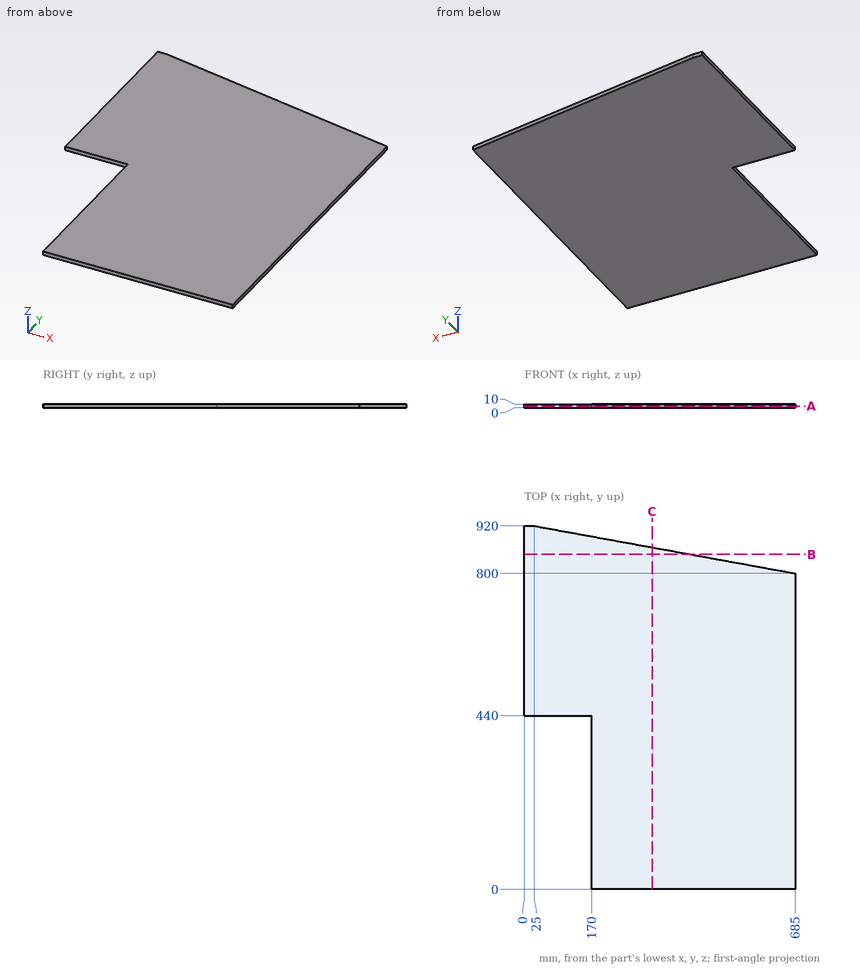
Can you work these out from the drawing? Everything is in mm from the part's minimum corner. Give positions to 0.01 mm unless a question says otherwise; leave off trailing zeros. Loops run counter-clockwise (first coordinate to the right, second up) from the corner with the lowest first, then second, coordinate; pieces in that order, holes last. Notation, with made-up numbers: (11, -31) -> (34, -31) arc R24 cw to (34, -21) -> close; hole circle Ø6 at (1.5, 15). An arc over 180 degrees is marked (long way). Return JSON: item names as keys, results as strings.
Q1. I want a section at C-C, the plane x = 323.5. List the corners of the cut face in (y, z) for me, then the cut area to 3 significant figures.
Checks:
{"outline": "(0, 0) -> (865.73, 0) -> (865.73, 10) -> (0, 10) -> close", "area": "8,660 mm2"}
Q2. I want a section at B-B, the plane y = 848. List the corners of the cut face in (x, z) for me, then the cut area to 3 significant figures.
Checks:
{"outline": "(0, 0) -> (421, 0) -> (421, 10) -> (0, 10) -> close", "area": "4,210 mm2"}
Q3. I need wall thicknesses on probe 1 along X at (y, z) = (134, 2.5); probe 2 along Y at (x, z) = (569, 4.25); probe 3 along Y at (x, z) = (196.5, 1.75). Which ranges of each line are inside material? Lowest first, please.
Checks:
{"probe 1": "x = 170 to 685", "probe 2": "y = 0 to 821.09", "probe 3": "y = 0 to 888.82"}
Q4. I want a section at A-A, the plane z = 4.5. List the corners of the cut face in (x, y) for me.
Checks:
{"outline": "(0, 440) -> (170, 440) -> (170, 0) -> (685, 0) -> (685, 800) -> (25, 920) -> (0, 920) -> close"}
Q5. For pin 1 Ø5 at (x, z) = (73, 3) entering from -Y; pin 2 Ø6 at (x, z) = (456, 2) entering from +Y; pin 3 Ø1.5 at (x, z) = (603.5, 6) entering from +Y, each with a flat end and sliding along its axis, tell me the tip position at first contact or that it passes through.
Checks:
{"pin 1": "stops at y = 440", "pin 2": "stops at y = 842.18", "pin 3": "stops at y = 814.95"}
